Can you work these out from the model? Positions are in its coordinate system, mm. A direction names the side the tool comes from. Round coordinates to 2 decimals unless told otherwise and drop trailing zeros. Loops run counter-clockwise (first coordinate to the right, second up) from the corner with the lowest first, then second, coordinate; pieces in that order, holes last. Notation, with made-up numbers: (-34.75, -28) -> (8.25, -28) arc R31 cw to (8.25, 8) -> close; hole circle Ø5 at (6, 3.5). An arc over 180 degrees is marked (long way). Write item = value, one per line.
from build123d import *

# Parameters (mm, degrees)
SKETCH_1_W      = 20.1
SKETCH_1_H      = 14
SKETCH_1_R      = 1
EXTRUDE_1_DEPTH = 2
SKETCH_2_W      = 10
SKETCH_2_H      = 14
EXTRUDE_2_DEPTH = 0.2
FILLET_1_R      = 2


with BuildPart() as part:
    # 草图1 → 凸台-拉伸1 (new body)
    with BuildSketch(Plane(origin=(0, 0, 0), x_dir=(1, 0, 0), z_dir=(0, 1, 0))):
        Rectangle(SKETCH_1_W, SKETCH_1_H)
        with Locations(Location((-8.05, 0, 0), (0, 0, 270))):
            Circle(SKETCH_1_R, mode=Mode.SUBTRACT)
        with Locations(Location((8.05, 0, 0), (0, 0, 90))):
            Circle(SKETCH_1_R, mode=Mode.SUBTRACT)
    extrude(amount=EXTRUDE_1_DEPTH)

    # 草图2 → 凸台-拉伸2 (add)
    with BuildSketch(Plane(origin=(0, 2, 0), x_dir=(1, 0, 0), z_dir=(0, 1, 0))):
        Rectangle(SKETCH_2_W, SKETCH_2_H)
    extrude(amount=EXTRUDE_2_DEPTH)

    # 圆角1
    fillet_1_edges = [part.edges().sort_by_distance(p)[0] for p in [
        (10.05, 1, 7),
        (-10.05, 1, 7),
        (-10.05, 1, -7),
        (10.05, 1, -7),
    ]]
    fillet(fillet_1_edges, radius=FILLET_1_R)


solid = part.part
1. Suppose I cut it at C-C, the plane z = 2. List the corners of the cut face in (x, y) for me.
Entries:
outline = (-10.05, 0) -> (10.05, 0) -> (10.05, 2) -> (5, 2) -> (5, 2.2) -> (-5, 2.2) -> (-5, 2) -> (-10.05, 2) -> close
2. Suppose I cut it at A-A, the plane z = 0. List the corners of the cut face in (x, y) for me.
Entries:
outline = (-10.05, 0) -> (-9.05, 0) -> (-9.05, 2) -> (-10.05, 2) -> close; (-7.05, 0) -> (7.05, 0) -> (7.05, 2) -> (5, 2) -> (5, 2.2) -> (-5, 2.2) -> (-5, 2) -> (-7.05, 2) -> close; (9.05, 0) -> (10.05, 0) -> (10.05, 2) -> (9.05, 2) -> close
3. I'm going to push a flat-ended pin straight in: pin 1 (3 mm diameter, centred on x = 8.05, z = 0, fed in from +Y). Where does the tip first touch, or does it pass through?
Entries:
pin_1 = 2
4. I need wall thicknesses on line 1 (X direction, y = 0.5, z = 0); line 2 (Z direction, x = 8.05, y = 1.3); line 3 (Y direction, x = 7.5, z = 1). Which ranges of each line are inside material? Lowest first, please. Write a range as [from, to].
Entries:
line_1 = [-10.05, -9.05], [-7.05, 7.05], [9.05, 10.05]
line_2 = [-7, -1], [1, 7]
line_3 = [0, 2]
5. Suppose I cut it at D-D, the plane x = 8.5. List the corners of the cut face in (y, z) for me.
Entries:
outline = (0, -6.95) -> (2, -6.95) -> (2, -0.89) -> (0, -0.89) -> close; (0, 0.89) -> (2, 0.89) -> (2, 6.95) -> (0, 6.95) -> close
6. Suppose I cut it at B-B, the plane y = 1.5. List the corners of the cut face in (x, z) for me.
Entries:
outline = (-10.05, -5) arc R2 ccw to (-8.05, -7) -> (8.05, -7) arc R2 ccw to (10.05, -5) -> (10.05, 5) arc R2 ccw to (8.05, 7) -> (-8.05, 7) arc R2 ccw to (-10.05, 5) -> close; hole circle Ø2 at (-8.05, 0); hole circle Ø2 at (8.05, 0)
7. We'd pull the mould along X, two halves only. Please class faces 4 (the cylindrical face through (9.45, 1.01, 6.43)), 5 (the cylindrical face through (-7.06, 0.99, -0.13)), 6 (the flat face through (0, 1, 7)): released by +X, released by -X, zero draft, split by the parting line, or undercut.
Entries:
face_4 = released by +X
face_5 = undercut
face_6 = zero draft
8. For faces 1 (the flat face through (6.9, 2, -0.1)), 2 (the flat face through (0, 2.2, 0)), 3 (the flat face through (-6, 2, 0)), which set-ups out of +Z, -Z, +X, -X, +Y, -Y let a thin tool reach every point of the face, with its end or its side?
Entries:
face_1 = +Z, -Z, +X, +Y
face_2 = +Z, -Z, +X, -X, +Y
face_3 = +Z, -Z, -X, +Y
